from build123d import *

# Parameters (mm, degrees)
BOSS_EXTRUDE1_DEPTH     = 101.6
SKETCH3_W               = 25.4
SKETCH3_H               = 101.6
BOSS_EXTRUDE2_DEPTH     = 50.8
CUT_EXTRUDE2_DEPTH      = 25.4
SKETCH6_R               = 3.2639
CUT_EXTRUDE3_DEPTH      = 101.6
SKETCH7_W               = 15.875
SKETCH7_H               = 7.928770879
CUT_EXTRUDE4_DEPTH      = 1
CUT_EXTRUDE4_DEPTH_BACK = 102.6


with BuildPart() as part:
    # Sketch2 → Boss-Extrude1 (new body)
    with BuildSketch(Plane(origin=(0, 0, 0), x_dir=(1, 0, 0), z_dir=(0, 1, 0))):
        Polygon((0, 2.159), (0, 0), (-3.937, 0), (0, -5.769770879), (6.35, -5.769770879), (10.287, 0), (6.35, 0), (6.35, 2.159), align=None)
    extrude(amount=-BOSS_EXTRUDE1_DEPTH)

    # Sketch3 → Boss-Extrude2 (add)
    with BuildSketch(Plane(origin=(0, 0, -2.159), x_dir=(-1, 0, 0), z_dir=(0, 0, -1))):
        with Locations((-3.175, -50.8)):
            Rectangle(SKETCH3_W, SKETCH3_H)
    extrude(amount=BOSS_EXTRUDE2_DEPTH)

    # Sketch5 → Cut-Extrude2 (cut)
    with BuildSketch(Plane(origin=(15.875, 0, 0), x_dir=(0, 0, -1), z_dir=(1, 0, 0))):
        with BuildLine():
            ThreePointArc((52.959, -88.9), (49.239256121, -97.880256121), (40.259, -101.6))
            Line((40.259, -101.6), (52.959, -101.6))
            Line((52.959, -101.6), (52.959, -88.9))
        make_face()
        with BuildLine():
            Line((52.959, 0), (40.259, 0))
            ThreePointArc((40.259, 0), (49.239256121, -3.719743879), (52.959, -12.7))
            Line((52.959, -12.7), (52.959, 0))
        make_face()
        with BuildLine():
            Line((40.259, -76.2), (40.259, -25.4))
            ThreePointArc((40.259, -25.4), (36.539256121, -16.419743879), (27.559, -12.7))
            Line((27.559, -12.7), (9.779, -12.7))
            Line((9.779, -12.7), (9.779, -88.9))
            Line((9.779, -88.9), (27.559, -88.9))
            ThreePointArc((27.559, -88.9), (36.539256121, -85.180256121), (40.259, -76.2))
        make_face()
    extrude(amount=-CUT_EXTRUDE2_DEPTH, mode=Mode.SUBTRACT)

    # Sketch6 → Cut-Extrude3 (cut)
    with BuildSketch(Plane(origin=(0, 0, 0), x_dir=(1, 0, 0), z_dir=(0, 1, 0))):
        with Locations((3.175, 17.399)):
            Circle(SKETCH6_R)
    extrude(amount=-CUT_EXTRUDE3_DEPTH, mode=Mode.SUBTRACT)

    # Sketch7 → Cut-Extrude4 (cut, two sides)
    with BuildSketch(Plane(origin=(0, 0, 0), x_dir=(1, 0, 0), z_dir=(0, 1, 0))) as cut_extrude4_sk:
        with Locations((3.175, -1.805385439)):
            Rectangle(SKETCH7_W, SKETCH7_H)
    extrude(amount=CUT_EXTRUDE4_DEPTH, mode=Mode.SUBTRACT)
    extrude(cut_extrude4_sk.sketch, amount=-CUT_EXTRUDE4_DEPTH_BACK, mode=Mode.SUBTRACT)


solid = part.part
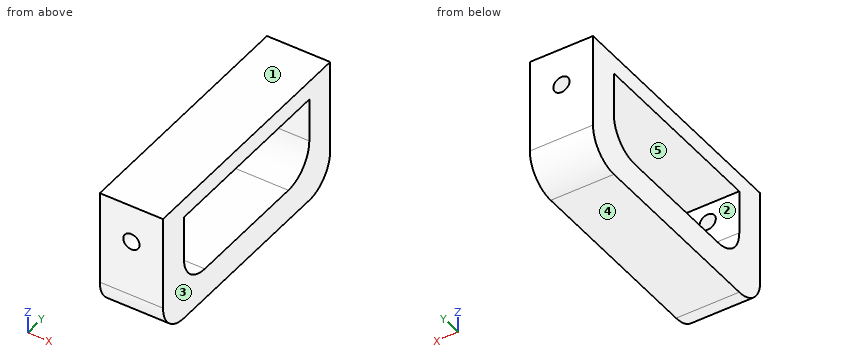
Read the model definition and answer for the solid it produces. Units are mm, in the model's axes. Face numbers are marked on the shaded views. A direction names the side the tool comes from. Give positions to 0.01 mm unless a question says otherwise; leave off trailing zeros. Write each loop counter-clockwise with the first axis right and the second up, starting at its lowest first coordinate (ties: lowest second). Pieces come first, ordered by that corner, then holes. Notation, with made-up numbers: (56, 28.5) - (111, 28.5) arc R15 ccw to (111, 41.5) - close; hole circle Ø2 at (61, 58). An arc over 180 degrees is marked (long way). Answer in a Markdown table with one row per item. Add a question column.
Item 1: Section C-C, the plane z = -12.5 is taken. Write down the section's boundary in (x, y) (3 decimals), and give its area (3 significant figures).
Item 2: Section A-A, the plane y = -32 is taken. Write down the section's boundary in (x, z) (3 decimals).
Item 3: Section D-D, the plane x = 1 is taken. Write down the section's boundary in (y, z), and give its area (3 significant figures).
Item 4: Flat-ended cylindrical pins translate along their axes: P1, Ø10.5, axis at x = 3.175, z = -17.399, coming from the +Y side; P2, Ø1, axis at x = 6, z = -45.5, coming from the +Y side. Find the tip coordinate at first contact, or state that the pin passes through.
Item 5: Section B-B, the plane x = 11.5 is taken. Write down the section's boundary in (y, z).
Item 6: A tool of negligible diameter and unlimited length cuts with its end or side. For the marked faces 4 and 5, from which of +Z, -Z, +X, -X, +Y, -Y can it reach the whole face along a straight path? Write none if from no direction.
Item 7: Find the intervals of material crossed by L1, parallel to Z at x = 11.5, y = -27; L2, parallel to Y at x = -4, z = -10; L3, parallel to X at y = -3.5, z = -16 (3 decimals), in increasing order.
Item 8: Determine the mould class of the marked faces 1, 2 and 3 for opening direction Z: pulls with the +Z half, pulls with the -Z half, needs draft (parallel to the pull), parting line crosses it, or undercut.
Recorded:
| question | item | result |
|---|---|---|
| 1 | outline | (-9.525, -101.6) - (15.875, -101.6) - (15.875, -88.9) - (-9.525, -88.9) - close; (-9.525, -12.7) - (15.875, -12.7) - (15.875, 0) - (-9.525, 0) - close |
| 1 | area | 645 mm2 |
| 2 | outline | (-9.525, -52.959) - (15.875, -52.959) - (15.875, -40.259) - (-9.525, -40.259) - close; (-9.525, -9.779) - (15.875, -9.779) - (15.875, -2.159) - (-9.525, -2.159) - close |
| 3 | outline | (-101.6, -40.26) arc R12.7 ccw to (-88.9, -52.96) - (-12.7, -52.96) arc R12.7 ccw to (0, -40.26) - (0, -19.83) - (-12.7, -19.83) - (-12.7, -27.56) arc R12.7 cw to (-25.4, -40.26) - (-76.2, -40.26) arc R12.7 cw to (-88.9, -27.56) - (-88.9, -19.83) - (-101.6, -19.83) - close; (-101.6, -14.97) - (-88.9, -14.97) - (-88.9, -9.78) - (-12.7, -9.78) - (-12.7, -14.97) - (0, -14.97) - (0, -2.16) - (-101.6, -2.16) - close |
| 3 | area | 2,720 mm2 |
| 4 | P1 | stops at y = 0 |
| 4 | P2 | stops at y = -0.92 |
| 5 | outline | (-101.6, -40.26) arc R12.7 ccw to (-88.9, -52.96) - (-12.7, -52.96) arc R12.7 ccw to (0, -40.26) - (0, -2.16) - (-101.6, -2.16) - close; hole (-88.9, -27.56) arc R12.7 ccw to (-76.2, -40.26) - (-25.4, -40.26) arc R12.7 ccw to (-12.7, -27.56) - (-12.7, -9.78) - (-88.9, -9.78) - close |
| 6 | face 4 | -Z, +X, -X, +Y, -Y |
| 6 | face 5 | +X, -X |
| 7 | L1 | z = -52.96 to -40.26, -9.78 to -2.16 |
| 7 | L2 | y = -101.6 to -88.9, -12.7 to 0 |
| 7 | L3 | x = -9.525 to 0.226, 6.124 to 15.875 |
| 8 | face 1 | pulls with the +Z half |
| 8 | face 2 | undercut |
| 8 | face 3 | needs draft |
